from build123d import *

# Parameters (mm, degrees)
F0_R           = 7.5
F1_DEPTH       = 25
F2_W           = 7.5
F2_H           = 45
F3_DEPTH       = 25
F5_D           = 5.5
F5_CBORE_D     = 9.75
F5_CBORE_DEPTH = 70
F6_R           = 20
F7_R           = 5
F8_R           = 10
F9_R           = 5
F11_DEPTH      = 100
F12_R          = 40


with BuildPart() as f1:
    # F0 (on Front) → F1 (new body)
    with BuildSketch(Plane.XZ):
        with BuildLine():
            Line((45.239401, 24.669705), (71.265909, -12.5))
            Line((71.265909, -12.5), (150, -12.5))
            Line((150, -12.5), (150, 62.5))
            Line((150, 62.5), (-12.5, 62.5))
            Line((-12.5, 62.5), (-12.5, 0))
            ThreePointArc((-12.5, 0), (0, -12.5), (12.5, 0))
            Line((12.5, 0), (23.776091, 23.002169))
            ThreePointArc((23.776091, 23.002169), (34.031763, 29.962444), (45.239401, 24.669705))
        make_face()
        Circle(F0_R, mode=Mode.SUBTRACT)
    extrude(amount=F1_DEPTH)

    # F2 (on Right) → F3 (cut, symmetric)
    with BuildSketch(Plane.YZ):
        with Locations((-3.75, -7.5)):
            Rectangle(F2_W, F2_H)
    extrude(amount=F3_DEPTH, both=True, mode=Mode.SUBTRACT)

    # F5 (through all)
    with Locations(Plane.XY.offset(62.5)):
        with Locations((140, -15), (115, -15), (90, -15)):
            CounterBoreHole(F5_D / 2, F5_CBORE_D / 2, F5_CBORE_DEPTH)

    # F6
    f6_edges = [f1.edges().sort_by_distance(p)[0] for p in [
        (-12.5, -12.5, 62.5),
    ]]
    fillet(f6_edges, radius=F6_R)

    # F7
    f7_edges = [f1.edges().sort_by_distance(p)[0] for p in [
        (3.676639, -7.5, 15),
    ]]
    fillet(f7_edges, radius=F7_R)

    # F8
    f8_edges = [f1.edges().sort_by_distance(p)[0] for p in [
        (150, -25, 25),
    ]]
    fillet(f8_edges, radius=F8_R)

    # F9
    f9_edges = [f1.edges().sort_by_distance(p)[0] for p in [
        (71.265909, -12.5, -12.5),
    ]]
    fillet(f9_edges, radius=F9_R)

    # F10 (on Top) → F11 (cut, symmetric)
    with BuildSketch(Plane.XY):
        Polygon((22.832396, -15), (-25, -15), (-25, -30), (55, -30), align=None)
    extrude(amount=F11_DEPTH, both=True, mode=Mode.SUBTRACT)

    # F12
    f12_edges = [f1.edges().sort_by_distance(p)[0] for p in [
        (22.832396, -15, 41.78856),
        (44.277465, -25, 44.188634),
    ]]
    fillet(f12_edges, radius=F12_R)


solid = f1.part
Model file for the job. Use its own axes, mm. A direction names the side the tool comes from. Give positions to 0.01 mm unless a question says otherwise; leave off trailing zeros. Loops run counter-clockwise (first coordinate to the right, second up) from the corner with the lowest first, then second, coordinate; pieces in that order, holes last.
Item 1: Slice it at C-C (z = -5.5). Write the cut outline in (x, y) (3 decimals), plus the area to 3 significant figures.
Check values:
outline: (-11.225, -15) - (-5.099, -15) - (-5.099, -7.5) - (-11.225, -7.5) - close; (5.099, -15) - (11.225, -15) - (11.225, -7.5) - (5.099, -7.5) - close; (66.364, -25) - (140, -25) arc R10 ccw to (150, -15) - (150, 0) - (66.364, 0) - close; hole circle Ø9.75 at (90, -15); hole circle Ø9.75 at (115, -15); hole circle Ø9.75 at (140, -15)
area: 1,940 mm2
Item 2: Drop flat-ended pins along their axis: P1, Ø5, axis at x = 115, y = -13.5, coming from the +Z side; P2, Ø7, axis at x = 3.5, z = -4.5, coming from the +Y side; P3, Ø5, axis at x = 140, y = -15, coming from the +Z side; P4, Ø10, axis at y = -21.5, z = 0, coming from the +X side. Give the stop position or say it passes through.
Check values:
P1: stops at z = -7.5
P2: stops at y = -7.5
P3: passes through
P4: stops at x = 149.89
Item 3: Slice it at A-A (x = 115). Write the cut outline in (y, z) (3 decimals), plus the area to 4 significant figures.
Check values:
outline: (-25, -12.5) - (-17.75, -12.5) - (-17.75, -7.5) - (-19.875, -7.5) - (-19.875, 62.5) - (-25, 62.5) - close; (-12.25, -12.5) - (0, -12.5) - (0, 62.5) - (-10.125, 62.5) - (-10.125, -7.5) - (-12.25, -7.5) - close
area: 1,165 mm2
Item 4: Mould opens along X. For faces 1 (the face through (110.13, -14.79, 27.99)), 2 (the face through (146.99, -22.15, 25.52)), 3 (the face through (80, -12, 62.5)) say: +X half, -X half, draft (parallel to the pull), parting line (faces both ways), or undercut.
Check values:
face 1: undercut
face 2: +X half
face 3: draft
Item 5: Slice it at B-B (z = 26.5). Write the cut outline in (x, y) (3 decimals), plus the area to 3 significant figures.
Check values:
outline: (-12.5, -15) - (13.965, -15) arc R40 cw to (26.325, -16.958) - (26.325, 0) - (-12.5, 0) - close; (43.675, -23.863) arc R40 ccw to (53.145, -25) - (140, -25) arc R10 ccw to (150, -15) - (150, 0) - (43.675, 0) - close; hole circle Ø9.75 at (90, -15); hole circle Ø9.75 at (115, -15); hole circle Ø9.75 at (140, -15)
area: 3,000 mm2
Item 6: Slice it at D-D (x = 5.5). Write the cut outline in (y, z), plus the area to 3 significant figures.
Check values:
outline: (-15, -11.22) - (-7.5, -11.22) - (-7.5, -5.1) - (-15, -5.1) - close; (-15, 5.1) - (-7.5, 5.1) - (-7.5, 10) arc R5 cw to (-2.5, 15) - (0, 15) - (0, 62.4) - (-15, 62.4) - close
area: 837 mm2
Item 7: Drill centre lines: line 1 along X through (y, z) = (-11.75, 18.5); line 2 along Y through (x, z) = (119, 6); line 3 along Y through (x, z) = (115, -8.8). Where is each one in solid material? Low to high.
Check values:
line 1: x = -12.5 to 21.57, 49.56 to 86.37, 93.63 to 111.37, 118.63 to 136.37, 143.63 to 150
line 2: y = -25 to -17.79, -12.21 to 0
line 3: y = -25 to -17.75, -12.25 to 0
Item 8: Which spindle directions (+Z, -Z, +X, -X, +Y, -Y) get a long thin tool onto all of the face, cutting with end or side? Do faces 4 (the face through (57.33, -12.33, 7.4)), 5 (the face through (44.61, -24.08, 43.74)), 6 (the face through (142.1, -17.1, -7.5)), 7 (the face through (6, -7.5, 6)). Say none if no direction does.
Check values:
face 4: -Z, +Y, -Y
face 5: +Z, -Z, -X, -Y
face 6: +Z
face 7: -Z, -X, +Y
